```python
from build123d import *

# Parameters (mm, degrees)
SKETCH1_R            = 11.500000000000002
SKETCH1_R_2          = 6.5
BOSS_EXTRUDE1_DEPTH  = 22
BOSS_EXTRUDE3_START  = 82
BOSS_EXTRUDE3_DEPTH  = 82
FILLET3_R            = 2.5
FILLET3_OF_MIRROR1_R = 2.5


with BuildPart() as part:
    # Sketch1 → Boss-Extrude1 (new body)
    # profile 1 of 3: a face of its own
    with BuildSketch(Plane(origin=(0, 0, 0), x_dir=(0, 0, -1), z_dir=(1, 0, 0))):
        Circle(SKETCH1_R)
        Circle(SKETCH1_R_2, mode=Mode.SUBTRACT)
    # profile 2 of 3: a face of its own
    with BuildSketch(Plane(origin=(0, 0, 0), x_dir=(0, 0, -1), z_dir=(1, 0, 0))):
        with BuildLine():
            Line((-11.5, 46), (-11.499999999999998, 5.047646745e-08))
            ThreePointArc((-11.500000000000002, 5.047646664e-08), (2.523823332e-08, 11.500000000000002), (11.500000000000002, 0))
            Line((11.500000000000002, 0), (11.499999999999998, 46))
            ThreePointArc((11.500000000000004, 46), (10.035533905932741, 42.46446609406726), (6.500000000000003, 41))
            Line((6.500000000000003, 41), (-6.499999999999997, 41))
            ThreePointArc((-6.499999999999998, 41), (-10.035533905932734, 42.46446609406726), (-11.499999999999996, 46))
        make_face()
    # profile 3 of 3: a face of its own
    with BuildSketch(Plane(origin=(0, 0, 0), x_dir=(0, 0, -1), z_dir=(1, 0, 0))):
        with BuildLine():
            Line((-11.5, 58.99999999999999), (-11.5, 46))
            ThreePointArc((-11.499999999999996, 46), (-10.035533905932734, 42.46446609406726), (-6.499999999999998, 41))
            Line((-6.499999999999997, 41), (6.500000000000003, 41))
            ThreePointArc((6.500000000000003, 41), (10.035533905932741, 42.46446609406726), (11.500000000000004, 46))
            Line((11.499999999999998, 46), (11.499999999999998, 59.00000000000001))
            ThreePointArc((11.499999999999998, 59.00000000000001), (10.035533905932727, 62.53553390593273), (6.5, 63.999999999999986))
            Line((6.5, 63.999999999999986), (-6.5, 64))
            ThreePointArc((-6.5, 64), (-10.035533905932738, 62.53553390593274), (-11.5, 59))
        make_face()
    boss_extrude1 = extrude(amount=-BOSS_EXTRUDE1_DEPTH)

    # Sketch1_4 → Boss-Extrude3 (add)
    with BuildSketch(Plane(origin=(0, 0, 0), x_dir=(0, 0, -1), z_dir=(1, 0, 0)).offset(BOSS_EXTRUDE3_START)):
        with BuildLine():
            Line((-11.5, 58.99999999999999), (-11.5, 46))
            ThreePointArc((-11.499999999999996, 46), (-10.035533905932734, 42.46446609406726), (-6.499999999999998, 41))
            Line((-6.499999999999997, 41), (6.500000000000003, 41))
            ThreePointArc((6.500000000000003, 41), (10.035533905932741, 42.46446609406726), (11.500000000000004, 46))
            Line((11.499999999999998, 46), (11.499999999999998, 59.00000000000001))
            ThreePointArc((11.499999999999998, 59.00000000000001), (10.035533905932727, 62.53553390593273), (6.5, 63.999999999999986))
            Line((6.5, 63.999999999999986), (-6.5, 64))
            ThreePointArc((-6.5, 64), (-10.035533905932738, 62.53553390593274), (-11.5, 59))
        make_face()
    extrude(amount=-BOSS_EXTRUDE3_DEPTH)

    # Fillet3
    fillet3_edges = [part.edges().sort_by_distance(p)[0] for p in [
        (0, 23.000000025238233, 11.5),
        (0, 23, -11.500000000000002),
        (-22, 62.53553390593273, -10.035533905932729),
        (-22, 63.99999999999999, 0),
        (-22, 62.53553390593274, 10.035533905932738),
        (-22, 29.500000025238233, 11.5),
        (-22, -11.500000000000002, 2.523822962e-08),
        (-22, 29.500000000000004, -11.500000000000002),
        (0, -11.500000000000002, 2.523822962e-08),
    ]]
    fillet(fillet3_edges, radius=FILLET3_R)

    # Mirror1: Boss-Extrude1 across plane
    add(boss_extrude1.mirror(Plane(origin=(41.00000000000001, 0, 0), x_dir=(0, 0, 1), z_dir=(1, 0, 0))))

    # Fillet3 of Mirror1
    fillet3_of_mirror1_edges = [part.edges().sort_by_distance(p)[0] for p in [
        (82.00000000000001, 23.000000025238233, 11.5),
        (82.00000000000001, 23, -11.500000000000002),
        (104.00000000000001, 62.53553390593273, -10.035533905932729),
        (104.00000000000001, 63.99999999999999, 0),
        (104.00000000000001, 62.53553390593274, 10.035533905932738),
        (104.00000000000001, 29.500000025238233, 11.5),
        (104.00000000000001, -11.500000000000002, 2.523822962e-08),
        (104.00000000000001, 29.500000000000004, -11.500000000000002),
        (82.00000000000001, -11.500000000000002, 2.523822962e-08),
    ]]
    fillet(fillet3_of_mirror1_edges, radius=FILLET3_OF_MIRROR1_R)


solid = part.part
```
Can you work these out from the model? Positions are in its coordinate system, mm. A direction names the side the tool comes from. Round coordinates to 2 decimals unless told otherwise and drop trailing zeros. Loops run counter-clockwise (first coordinate to the right, second up) from the corner with the lowest first, then second, coordinate; pieces in that order, holes last. Notation, with made-up numbers: (-5, 42.5) -> (9, 42.5) arc R23 cw to (9, 74.5) -> close; hole circle Ø10 at (-15, 56). An arc over 180 degrees is marked (long way). One line per item, written item: value. Start each with the question number.
1. If I drill on probe 1 along X at (y, z) = (-3, -6.5); probe 2 along Y at (x, z) = (87.5, 0); probe 3 along Y at (x, z) = (69, -4.5), over which ranges is the centre line in solid material (lowest first)?
2. For faces 1 (the cylindrical face through (41.61, 42.43, -10)), 2 (the flat face through (40, 49, -11.5)), 3 (the cylindrical face through (41.61, 42.5, 10.07)), which set-ups out of +Z, -Z, +X, -X, +Y, -Y let a thin tool reach every point of the face, with its end or its side?
3. If we mould it in two halves opening along X, with no side actions, what happens to faces 4 (the cylindrical face through (-21.248, 63.287, 0.091)), 5 (the cylindrical face through (83, 23, 11)), 6 (the flat face through (40, 64, 0))? For each: pulls with the +X half, pulls with the -X half, needs draft (parallel to the pull), parting line crosses it, or undercut.
4. For pin 1 (1 mm diameter, centred on x = 5.5, z = -6.5, fed in from -Y); pin 2 (1.5 mm diameter, centred on x = 24, y = 41.5, fed in from +Z), each with a flat end and sliding along its axis, tell me the tip position at first contact or that it passes through.
5. If we section it at B-B, the plane x = 59: Write out the boundary of the cut face in (y, z).
6. If we section it at A-A, the plane z = 0: Write out the boundary of the cut face in (x, y).
Calculated:
1. probe 1: x = -22 to 0, 82 to 104
1. probe 2: y = -11.5 to -6.5, 6.5 to 64
1. probe 3: y = 41 to 64
2. face 1: -Z, -Y
2. face 2: -Z, +X, -X, +Y, -Y
2. face 3: +Z, -Y
3. face 4: pulls with the -X half
3. face 5: undercut
3. face 6: needs draft
4. pin 1: stops at y = 41
4. pin 2: stops at z = 9.81
5. outline: (41, -6.5) arc R5 ccw to (46, -11.5) -> (59, -11.5) arc R5 ccw to (64, -6.5) -> (64, 6.5) arc R5 ccw to (59, 11.5) -> (46, 11.5) arc R5 ccw to (41, 6.5) -> close
6. outline: (-22, -9) arc R2.5 ccw to (-19.5, -11.5) -> (-2.5, -11.5) arc R2.5 ccw to (0, -9) -> (0, -6.5) -> (-22, -6.5) -> close; (-22, 6.5) -> (0, 6.5) -> (0, 41) -> (82, 41) -> (82, 6.5) -> (104, 6.5) -> (104, 61.5) arc R2.5 ccw to (101.5, 64) -> (-19.5, 64) arc R2.5 ccw to (-22, 61.5) -> close; (82, -9) arc R2.5 ccw to (84.5, -11.5) -> (101.5, -11.5) arc R2.5 ccw to (104, -9) -> (104, -6.5) -> (82, -6.5) -> close
